from build123d import *

# Parameters (mm, degrees)
SKETCH1_R           = 31.75
SKETCH1_R_2         = 13.788571429
BOSS_EXTRUDE1_DEPTH = 20.32
CUT_EXTRUDE1_DEPTH  = 13.97
SKETCH13_R          = 31.75
SKETCH13_R_2        = 25
CUT_EXTRUDE2_DEPTH  = 10.16
CIRPATTERN1_COUNT   = 2


with BuildPart() as part:
    # Sketch1 → Boss-Extrude1 (new, symmetric)
    with BuildSketch(Plane(origin=(0, 0, 0), x_dir=(1, 0, 0), z_dir=(0, 1, 0))):
        with Locations(Location((0, 0, 0), (0, 0, 270))):
            Circle(SKETCH1_R)
        with Locations(Location((0, 0, 0), (0, 0, 270))):
            Circle(SKETCH1_R_2, mode=Mode.SUBTRACT)
    extrude(amount=BOSS_EXTRUDE1_DEPTH, both=True)

    # Sketch2 → Cut-Extrude1 (cut)
    with BuildSketch(Plane(origin=(0, 20.32, 0), x_dir=(1, 0, 0), z_dir=(0, 1, 0))):
        with BuildLine():
            Line((-20.066, 0), (-20.066, 24.60524627))
            ThreePointArc((-20.066, 24.60524627), (-18.088933462, 26.093159759), (-16.002, 27.422590979))
            Line((-16.002, 27.422590979), (-16.002, 12.107037292))
            ThreePointArc((-16.002, 12.107037292), (19.022887373, -6.385460986), (-20.066, 0))
        make_face()
    cut_extrude1 = extrude(amount=-CUT_EXTRUDE1_DEPTH, mode=Mode.SUBTRACT)

    # Sketch13 → Cut-Extrude2 (cut)
    with BuildSketch(Plane(origin=(0, 20.32, 0), x_dir=(1, 0, 0), z_dir=(0, 1, 0))):
        with Locations(Location((0, 0, 0), (0, 0, 120.264992611))):
            Circle(SKETCH13_R)
        Circle(SKETCH13_R_2, mode=Mode.SUBTRACT)
    cut_extrude2 = extrude(amount=-CUT_EXTRUDE2_DEPTH, mode=Mode.SUBTRACT)

    # CirPattern1: Cut-Extrude1, Cut-Extrude2 ×2 about axis
    cirpattern1_axis = Axis((0, 0, 0), (0, 0, 1))
    add([cut_extrude1.rotate(cirpattern1_axis, i * 360 / CIRPATTERN1_COUNT) for i in range(1, CIRPATTERN1_COUNT)], mode=Mode.SUBTRACT)
    add([cut_extrude2.rotate(cirpattern1_axis, i * 360 / CIRPATTERN1_COUNT) for i in range(1, CIRPATTERN1_COUNT)], mode=Mode.SUBTRACT)


solid = part.part
Can you work these out from the model? Positions are in its coordinate system, mm. A direction names the side the tool comes from. Round coordinates to 2 decimals unless told otherwise and drop trailing zeros. Loops run counter-clockwise (first coordinate to the right, second up) from the corner with the lowest first, then second, coordinate; pieces in that order, holes last. Notation, with made-up numbers: (82.5, 60.5) - (110.5, 60.5) arc R25 cw to (110.5, 88.5) - close; hole circle Ø5 at (-16, 62.25). An arc over 180 degrees is marked (long way). Write item = value, one per line. Start each with the question number.
(1) If we mould it in two halves opening along Z, with no side actions, what happens to faces 1 (the face through (-16.002, 12, -16)), 2 (the face through (19.26, 13.43, 5.63)), 3 (the face through (9.537, 0.142, 30.284))? For each: released by +Z, released by -Z, zero draft, split by the parting line, or undercut.
(2) If we section it at D-D (z = 21): Please give me the cut outline in (x, y).
(3) For P1, Ø5, axis at x = -17.5, y = -1, coming from the -Z side; P2, Ø10, axis at x = -7, y = -2.5, coming from the -Z side; P3, Ø10, axis at y = 6, z = 19.5, coming from the +X side, each with a flat end and sliding along its axis, tell me the tip position at first contact or that it passes through.
(4) For faces 4 (the face through (24, 10.16, 8)), 5 (the face through (-20.066, 13, -9)), 6 (the face through (0, -6.35, -15)), 7 (the face through (-5.281, -0.089, 12.737)), 8 (the face through (20.066, -13, -9)), which set-ups out of +Z, -Z, +X, -X, +Y, -Y let a thin tool reach every point of the face, with its end or its side?
(5) If we section it at C-C (y = 1): Please give me the cut outline in (x, z), and give its area (3 significant figures).
(6) If we section it at B-B (z = 5): Please give me the cut outline in (x, y), and give its area (3 significant figures).
(7) If we section it at A-A (x = 0): Please give me the cut outline in (y, z).
(8) If I drill on probe 1 along Z at (x, y) = (0, -10); probe 2 along Z at (x, y) = (0, 0), over which ranges is the centre line in solid material (lowest first)? Write a range as [from, to].
Ans:
q1.face_1 = zero draft
q1.face_2 = undercut
q1.face_3 = split by the parting line
q2.outline = (-23.81, -10.16) - (-13.56, -10.16) - (-13.56, -20.32) - (13.56, -20.32) - (13.56, -10.16) - (23.81, -10.16) - (23.81, 10.16) - (13.56, 10.16) - (13.56, 20.32) - (-13.56, 20.32) - (-13.56, 10.16) - (-23.81, 10.16) - close
q3.P1 = -27.98
q3.P2 = -31.69
q3.P3 = 28.25
q4.face_4 = +Y
q4.face_5 = -Z, +Y
q4.face_6 = -Y
q4.face_7 = +Y, -Y
q4.face_8 = -Z, -Y
q5.outline = circle Ø63.5 at (0, 0); hole circle Ø27.58 at (0, 0)
q5.area = 2,570 mm²
q6.outline = (-31.35, -10.16) - (-24.49, -10.16) - (-24.49, -20.32) - (-19.43, -20.32) - (-19.43, -6.35) - (-12.85, -6.35) - (-12.85, 6.35) - (-19.43, 6.35) - (-19.43, 20.32) - (-24.49, 20.32) - (-24.49, 10.16) - (-31.35, 10.16) - close; (12.85, -6.35) - (19.43, -6.35) - (19.43, -20.32) - (24.49, -20.32) - (24.49, -10.16) - (31.35, -10.16) - (31.35, 10.16) - (24.49, 10.16) - (24.49, 20.32) - (19.43, 20.32) - (19.43, 6.35) - (12.85, 6.35) - close
q6.area = 857 mm²
q7.outline = (-20.32, -25) - (-10.16, -25) - (-10.16, -31.75) - (10.16, -31.75) - (10.16, -25) - (20.32, -25) - (20.32, -20.07) - (6.35, -20.07) - (6.35, -13.79) - (-6.35, -13.79) - (-6.35, -20.07) - (-20.32, -20.07) - close; (-20.32, 20.07) - (-6.35, 20.07) - (-6.35, 13.79) - (6.35, 13.79) - (6.35, 20.07) - (20.32, 20.07) - (20.32, 25) - (10.16, 25) - (10.16, 31.75) - (-10.16, 31.75) - (-10.16, 25) - (-20.32, 25) - close
q8.probe_1 = [-31.75, -20.07], [20.07, 31.75]
q8.probe_2 = [-31.75, -13.79], [13.79, 31.75]
